Here's how the part is built. I have some questions about the finished solid (model axes, mm). A direction names the side the tool comes from. Give positions to 0.01 mm unless a question says otherwise; leave off trailing zeros. Order: outer loops, then holes, each group sorted by start corner. A loop starts at its lowest first (then second) coordinate and runs counter-clockwise, first axis right, second up. Notation, with made-up numbers: M 22.5,75 L 52.5,75 A24 cw 52.5,85 Z; hole C 27.25,33 d4. An arc over 180 degrees is marked long. Use one line per item in the form item = value.
from build123d import *

# Parameters (mm, degrees)
F0_R     = 6.7521335394
F0_R_2   = 6.8163388515
F1_DEPTH = 12.7
F2_R     = 6.7521335394
F3_DEPTH = 25.4
F5_DEPTH = 12.7


# Not quite as in the source:
# - a length typed as a fraction of an inch, garbled in the dataset ("3 / 203.2 mm" for 3/8 in), is restored


with BuildPart() as f1:
    # F0 (on Front) → F1 (new body)
    with BuildSketch(Plane.XZ):
        with BuildLine():
            ThreePointArc((-6.6273338161, 39.4025146961), (-27.5938108098, 60.3689916898), (-48.5602878034, 39.4025146961))
            Line((-48.5602878034, 39.4025146961), (-48.5602878034, -46.63233459))
            ThreePointArc((-48.5602878034, -46.63233459), (-27.5938108098, -67.5988115836), (-6.6273338161, -46.63233459))
            Line((-6.6273338161, -46.63233459), (-6.6273338161, 39.4025146961))
        make_face()
        with Locations((-27.5938108098, -46.63233459)):
            Circle(F0_R, mode=Mode.SUBTRACT)
        with Locations((-27.5938108098, 39.4025146961)):
            Circle(F0_R_2, mode=Mode.SUBTRACT)
    extrude(amount=F1_DEPTH)

    # F2 (on face) → F3 (join)
    with BuildSketch(Plane(origin=(0, 0, 0), x_dir=(-1, 0, 0), z_dir=(0, 1, 0))):
        with BuildLine():
            ThreePointArc((6.6273338161, -46.63233459), (27.5938108098, -67.5988115836), (48.5602878034, -46.63233459))
            ThreePointArc((48.5602878034, -46.63233459), (27.5938108098, -25.6658575963), (6.6273338161, -46.63233459))
        make_face()
        with Locations((27.5938108098, -46.63233459)):
            Circle(F2_R, mode=Mode.SUBTRACT)
    extrude(amount=F3_DEPTH)

    # F4 (on face) → F5 (join)
    with BuildSketch(Plane(origin=(0, 25.4, 0), x_dir=(-1, 0, 0), z_dir=(0, 1, 0))):
        with BuildLine():
            Line((6.6871955224, -45.0491116899), (6.6871955224, -48.21555749))
            Line((6.6871955224, -48.21555749), (20.5757935859, -48.21555749))
            ThreePointArc((20.5757935859, -48.21555749), (20.6464307387, -47.1868562222), (20.8570162136, -46.1774654835))
            ThreePointArc((20.8570162136, -46.1774654835), (25.5313250881, -40.2029131555), (32.8088623121, -42.3434483519))
            ThreePointArc((32.8088623121, -42.3434483519), (34.8864096094, -44.9587614977), (35.6275880547, -48.21555749))
            Line((35.6275880547, -48.21555749), (48.5004260971, -48.21555749))
            ThreePointArc((48.5004260971, -48.21555749), (48.545317032, -47.4245116811), (48.5602878034, -46.63233459))
            ThreePointArc((48.5602878034, -46.63233459), (28.385987901, -25.6808283677), (6.6871955224, -45.0491116899))
        make_face()
        with BuildLine():
            Line((6.6871955224, 42.21310094), (6.6871955224, -45.0491116899))
            ThreePointArc((6.6871955224, -45.0491116899), (28.385987901, -25.6808283677), (48.5602878034, -46.63233459))
            ThreePointArc((48.5602878034, -46.63233459), (48.545317032, -47.4245116811), (48.5004260971, -48.21555749))
            Line((48.5004260971, -48.21555749), (49.5161861181, -48.21555749))
            Line((49.5161861181, -48.21555749), (49.5161861181, 42.21310094))
            Line((49.5161861181, 42.21310094), (36.0246261847, 42.21310094))
            ThreePointArc((36.0246261847, 42.21310094), (28.1016908203, 34.2901655755), (20.1787554558, 42.21310094))
            Line((20.1787554558, 42.21310094), (6.6871955224, 42.21310094))
        make_face()
        with BuildLine():
            Line((20.5757935859, -48.21555749), (6.6871955224, -48.21555749))
            ThreePointArc((6.6871955224, -48.21555749), (17.4268777521, -64.4696352981), (36.8849828604, -65.427740397))
            ThreePointArc((36.8849828604, -65.427740397), (44.9731491209, -58.3605807245), (48.5004260971, -48.21555749))
            Line((48.5004260971, -48.21555749), (35.6275880547, -48.21555749))
            ThreePointArc((35.6275880547, -48.21555749), (28.1016908203, -55.7414547244), (20.5757935859, -48.21555749))
        make_face()
        with BuildLine():
            ThreePointArc((49.5161861181, 42.21310094), (28.1016908203, 63.6275962378), (6.6871955224, 42.21310094))
            Line((6.6871955224, 42.21310094), (20.1787554558, 42.21310094))
            ThreePointArc((20.1787554558, 42.21310094), (28.1016908203, 50.1360363044), (36.0246261847, 42.21310094))
            Line((36.0246261847, 42.21310094), (49.5161861181, 42.21310094))
        make_face()
    extrude(amount=F5_DEPTH)


solid = f1.part
Q1. I want a section at D-D on z = 44.5. Write out the boundary of the cut face in (x, y).
Found:
outline = M -49.39,25.4 L -35.69,25.4 L -35.69,38.1 L -49.39,38.1 Z; M -47.93,-12.7 L -32.12,-12.7 L -32.12,0 L -47.93,0 Z; M -23.07,-12.7 L -7.26,-12.7 L -7.26,0 L -23.07,0 Z; M -20.52,25.4 L -6.81,25.4 L -6.81,38.1 L -20.52,38.1 Z
Q2. I want a section at A-A on z = 9. Write out the boundary of the cut face in (x, y).
Found:
outline = M -49.52,25.4 L -6.69,25.4 L -6.69,38.1 L -49.52,38.1 Z; M -48.56,-12.7 L -6.63,-12.7 L -6.63,0 L -48.56,0 Z
Q3. On a 3-axis mill with a long thin cutter (end or side, diameter ignored), from which of +Z, -Z, +X, -X, +Y, -Y can I reach the whole of each face in a straight line? I mean faces 1 (the face through (-28.6, 25.4, -53.5)), 2 (the face through (-18, 25.4, -65)), 3 (the face through (-27.133, -6.261, 60.364)). Say none if no direction works.
Found:
face_1 = +Y
face_2 = -Z, +Y
face_3 = +Z, -Y
Q4. I want a section at C-C on x = -26. Write out the boundary of the cut face in (y, z), then the cut area to 3 significant figures.
Found:
outline = M -12.7,-67.54 L 25.4,-67.54 L 25.4,-67.2 L 38.1,-67.2 L 38.1,-55.44 L 25.4,-55.44 L 25.4,-53.19 L -12.7,-53.19 Z; M -12.7,-40.07 L 38.1,-40.07 L 38.1,34.57 L 25.4,34.57 L 25.4,-25.73 L 0,-25.73 L 0,32.78 L -12.7,32.78 Z; M -12.7,46.03 L 0,46.03 L 0,60.31 L -12.7,60.31 Z; M 25.4,49.85 L 38.1,49.85 L 38.1,63.52 L 25.4,63.52 Z
area = 3,290 mm²
Q5. I want a section at B-B on y = 29. Write out the boundary of the cut face in (x, z).
Found:
outline = M -49.52,-48.22 L -48.5,-48.22 A20.97 ccw -36.88,-65.43 A21.56 ccw -6.69,-48.22 L -6.69,42.21 A21.41 ccw -49.52,42.21 Z; hole C -28.1,42.21 d15.85; hole M -32.81,-42.34 A7.53 ccw long -20.86,-46.18 A6.75 ccw Z
Q6. I need wall thicknesses on L1, parallel to Z at x = -27, y = -1; L2, parallel to Y at x = -24.5, z = -1.5; L3, parallel to Z at x = -27.5, y = 10. Which ranges of each line are inside material? Lowest first, please.
Found:
L1 = -67.59 to -53.36, -39.91 to 32.61, 46.19 to 60.36
L2 = -12.7 to 0, 25.4 to 38.1
L3 = -67.6 to -53.38, -39.88 to -25.67
Q7. Thinking about a two-plate mould opening in X: for faces 4 (the face through (-48.56, -6, -3)), 5 (the face through (-28, 0, 8)), 6 (the face through (-33, -6.26, 35.25)), 7 (the face through (-34.389, 31.661, 37.392)), which applies, +X half, -X half, draft (parallel to the pull), parting line (faces both ways), or undercut?
Found:
face_4 = -X half
face_5 = draft
face_6 = undercut
face_7 = undercut
Q8. I'm going to push flat-ended pins straight in: pin 1 Ø14 at (y, z) = (-4.5, 17.5) entering from -X; pin 2 Ø1.5 at (x, y) = (-30.5, 21.5) entering from -Z; pin 3 Ø12 at (x, y) = (-26, 10.5) entering from -Z; pin 4 Ø14.5 at (x, z) = (-27, -47.5) entering from +Y. Where does each tip first touch, or does it pass through?
Found:
pin_1 = -48.56
pin_2 = -67.49
pin_3 = -67.6
pin_4 = 38.1
